Here's how the part is built. I have some questions about the finished solid (model axes, mm). A direction names the side the tool comes from. Round coordinates to 2 decimals unless told otherwise and drop trailing zeros. Loops run counter-clockwise (first coordinate to the right, second up) from the corner with the lowest first, then second, coordinate; pieces in that order, holes last. Notation, with made-up numbers: M 60,85.25 L 103,85.25 A25 cw 103,105.25 Z; hole C -7,54 d9. An arc over 180 degrees is marked long. Answer as a JSON object with one key per item and string values.
from build123d import *

# Parameters (mm, degrees)
BOSS_EXTRUDE1_DEPTH = 7
SKETCH2_W           = 12.012879562
SKETCH2_H           = 7
BOSS_EXTRUDE3_DEPTH = 5
CUT_EXTRUDE1_DEPTH  = 33.388269627
SKETCH4_R           = 1.2
CUT_EXTRUDE2_DEPTH  = 33.388269627


with BuildPart() as part:
    # Sketch1 → Boss-Extrude1 (new body)
    with BuildSketch(Plane(origin=(0, 0, 0), x_dir=(1, 0, 0), z_dir=(0, 1, 0))):
        with BuildLine():
            add(Edge.make_bspline(
                [(0, 11.802718513), (1.58072242, 5.981279649), (4.167222532, -0.050595561), (5, -4.726791588)],
                knots=[0.482657311, 0.482657311, 0.482657311, 0.482657311, 0.853883687, 0.853883687, 0.853883687, 0.853883687], degree=3))
            Line((0, 11.802718513), (5, 17.987120438))
            Line((5, 17.987120438), (5, 30))
            Line((5, 30), (-5, 30))
            Line((-5, 30), (-5, -30))
            Line((-5, -30), (5, -30))
            Line((5, -30), (5, -4.726791588))
        make_face()
    extrude(amount=BOSS_EXTRUDE1_DEPTH)

    # Sketch2 → Boss-Extrude3 (add)
    with BuildSketch(Plane(origin=(5, 0, 0), x_dir=(0, 0, -1), z_dir=(1, 0, 0))):
        with Locations((23.993560219, 3.5)):
            Rectangle(SKETCH2_W, SKETCH2_H)
    extrude(amount=BOSS_EXTRUDE3_DEPTH)

    # Sketch3 → Cut-Extrude1 (cut, through all)
    with BuildSketch(Plane(origin=(0, 7, 0), x_dir=(1, 0, 0), z_dir=(0, 1, 0))):
        Polygon((10, 28.05876983), (4.315561677, 23.993560219), (10, 19.0964891), align=None)
    extrude(amount=-CUT_EXTRUDE1_DEPTH, mode=Mode.SUBTRACT)

    # Sketch4 → Cut-Extrude2 (cut, through all)
    with BuildSketch(Plane(origin=(0, 7, 0), x_dir=(1, 0, 0), z_dir=(0, 1, 0))):
        with Locations(Location((0, -22.059676008, 0), (0, 0, 270))):
            Circle(SKETCH4_R)
        with Locations(Location((0, -18.059676008, 0), (0, 0, 270))):
            Circle(SKETCH4_R)
    extrude(amount=-CUT_EXTRUDE2_DEPTH, mode=Mode.SUBTRACT)


solid = part.part
Item 1: Please list where these lines run through material, in increasing order: probe 1 along Z at (x, y) = (-1, 5); probe 2 along X at (y, z) = (0.5, 14); probe 3 along Z at (x, y) = (7.75, 6.5). Write a range as from..to.
Resolved:
{"probe 1": "-30..17.4, 18.72..21.4, 22.72..30", "probe 2": "-5..5", "probe 3": "-30..-26.45, -21.03..-17.99"}
Item 2: I want a section at B-B, the plane z = 16. Please give me the cut outline in (x, y), then the cut area to 3 significant figures.
Resolved:
{"outline": "M -5,0 L 5,0 L 5,7 L -5,7 Z", "area": "70.0 mm²"}
Item 3: I want a section at C-C, the plane y = 5.75. State how many separate pieces and enclosed holes the cut face has, then the cut area to 3 significant figures.
Resolved:
{"separate pieces": "1", "enclosed holes": "2", "area": "570 mm²"}
Item 4: I want a section at D-D, the plane x = 6. Please give me the cut outline in (y, z), then the cut area to 3 significant figures.
Resolved:
{"outline": "M 0,-30 L 7,-30 L 7,-25.2 L 0,-25.2 Z; M 0,-22.54 L 7,-22.54 L 7,-17.99 L 0,-17.99 Z", "area": "65.5 mm²"}
Item 5: On a 3-axis mill with a long thin cutter (end or side, diameter ignored), from which of +Z, -Z, +X, -X, +Y, -Y can I reach the whole of each face in a straight line? I mean faces 5 (the face through (5, 3, 18)), 6 (the face through (10, 4, -29)), 7 (the face through (7.12, 3.55, -21.58)). Say none if no direction works.
Resolved:
{"face 5": "+Z, +X, +Y, -Y", "face 6": "+Z, -Z, +X, +Y, -Y", "face 7": "+X, +Y, -Y"}
Item 6: I'm going to push flat-ended pins straight in: pin 1 Ø4 at (x, y) = (7.5, 4.5) entering from +Z; pin 2 Ø2 at (y, z) = (3.5, 23.5) entering from +X. Where does each tip first touch, or does it pass through?
Resolved:
{"pin 1": "z = -17.99", "pin 2": "x = 5"}
Item 7: I want a section at A-A, the plane x = 8.5. Please give me the cut outline in (y, z), then the cut area to 3 significant figures.
Resolved:
{"outline": "M 0,-30 L 7,-30 L 7,-26.99 L 0,-26.99 Z; M 0,-20.39 L 7,-20.39 L 7,-17.99 L 0,-17.99 Z", "area": "37.9 mm²"}
Item 8: If we mould it in two halves opening along X, with no side actions, what happens to faces 1 (the face through (-5, 3, 0)), 2 (the face through (0.05, 3.55, 20.86)), 3 (the face through (0.36, 3.549, 19.204)), 4 (the face through (2, 3, -30))? For each: pulls with the +X half, pulls with the -X half, needs draft (parallel to the pull), parting line crosses it, or undercut.
Resolved:
{"face 1": "pulls with the -X half", "face 2": "undercut", "face 3": "undercut", "face 4": "needs draft"}
